Read the model definition and answer for the solid it produces. Units are mm, in the model's axes. A direction names the side the tool comes from. Give positions to 0.01 mm unless a question says otherwise; leave off trailing zeros. Write each loop counter-clockwise with the first axis right and the second up, starting at its lowest first coordinate (ties: lowest second). Pieces come first, ordered by that corner, then holes. Notation, with made-up numbers: (42, 9.25) -> (89, 9.25) arc R12 ccw to (89, 18.25) -> close; hole circle Ø4 at (-23.75, -7). An arc over 180 degrees is marked (long way). Answer as CSV lines item,"result". Start each with the question number.
1. Given pin 1 (1.6 mm diameter, centred on x = 0, y = 0, fed in from -Z); pin 2 (2 mm diameter, centred on y = -1.5, z = 12, fed in from +X), each flat-ended and moving along its own axis, determine where each tip first touches the part or whether it passes through.
2. Find the intervals of material crossed by line 1 (Y direction, x = 0, z = 3.25); line 2 (Z direction, x = 0, y = 1.5); line 3 (Z direction, x = 0, y = -1.7), in increasing order.
3. For a pull along Z with two mould halves and no side action, classify faces 1 (the flat face through (7, -3, 18)), 2 (the cylindrical face through (0.846, 0.042, 23.945)), 3 (the flat face through (0, -2, 0)) as pulls with the +Z half, pulls with the -Z half, needs draft (parallel to the pull), parting line crosses it, or undercut.
4. A tool of negligible diameter and unlimited length cuts with its end or side. For faces 4 (the cylindrical face through (-0.54, -2.44, 4.93)), 5 (the cylindrical face through (6.64, -0.04, 24.1)), from which of +Z, -Z, +X, -X, +Y, -Y can it reach the whole face along a straight path? Write none if from no direction.
5. The part is cut by section A-A, the plane x = 0. Determine the outline of the cut face in (y, z).
6. The part is cut by section C-C, the plane y = 0. Determine the outline of the cut face in (x, z), and give its area (3 significant figures).
7. The part is cut by section D-D, the plane z = 3.5. Determine the outline of the cut face in (x, y).
8. The part is cut by section B-B, the plane z = 17.5. Determine the outline of the cut face in (x, y).
from build123d import *

# Parameters (mm, degrees)
SKETCH_R        = 2.5
PAD_DEPTH       = 20
SKETCH001_R     = 1.6
POCKET_DEPTH    = 10
POCKET_FACE3_R  = 2.5
POCKET001_DEPTH = 10
SKETCH002_W     = 15
SKETCH002_H     = 15
PAD001_DEPTH    = 3
PAD002_DEPTH    = 3
SKETCH003_R     = 6.5
POCKET002_DEPTH = 6.001
FILLET_R        = 3


with BuildPart() as part:
    # Sketch → Pad (new body)
    with BuildSketch(Plane.XY):
        Circle(SKETCH_R)
    extrude(amount=PAD_DEPTH)

    # Sketch001 (on Face2 of Pad) → Pocket (cut)
    with BuildSketch(Plane(origin=(0, 0, 0), x_dir=(1, 0, 0), z_dir=(0, 0, -1))):
        Circle(SKETCH001_R)
    extrude(amount=-POCKET_DEPTH, mode=Mode.SUBTRACT)

    # Pocket Face3 → Pocket001 (cut)
    with BuildSketch(Plane(origin=(0, 0, 20), x_dir=(0, 1, 0), z_dir=(0, 0, 1))):
        Circle(POCKET_FACE3_R)
    extrude(amount=-POCKET001_DEPTH, mode=Mode.SUBTRACT)

    # Sketch002 → Pad001 (join)
    with BuildSketch(Plane.XZ):
        with Locations((0, 17.5)):
            Rectangle(SKETCH002_W, SKETCH002_H)
    extrude(amount=PAD001_DEPTH)

    # Pad001 Face5 → Pad002 (add)
    with BuildSketch(Plane(origin=(0, 0, 17.5), x_dir=(1, 0, 0), z_dir=(0, 1, 0))):
        Polygon((7.5, -7.5), (7.5, 7.5), (2.5, 7.5), (1.6, 7.5), (-1.6, 7.5), (-2.5, 7.5), (-7.5, 7.5), (-7.5, -7.5), align=None)
    extrude(amount=PAD002_DEPTH)

    # Sketch003 (on Face3 of Pad002) → Pocket002 (cut, through all)
    with BuildSketch(Plane(origin=(0, 3, 0), x_dir=(-1, 0, 0), z_dir=(0, 1, 0))):
        with Locations((0, 17.5)):
            Circle(SKETCH003_R)
    extrude(amount=-POCKET002_DEPTH, mode=Mode.SUBTRACT)

    # Fillet
    fillet_edges = [part.edges().sort_by_distance(p)[0] for p in [
        (-7.5, 0, 25),
        (-7.5, 0, 10),
        (7.5, 0, 25),
        (7.5, 0, 10),
    ]]
    fillet(fillet_edges, radius=FILLET_R)


solid = part.part
Results found:
1,pin 1,"stops at z = 10"
1,pin 2,"stops at x = 7.5"
2,line 1,"y = -2.5 to -1.6, 1.6 to 2.5"
2,line 2,"z = 10 to 11, 24 to 25"
2,line 3,"z = 0 to 11, 24 to 25"
3,face 1,"needs draft"
3,face 2,"undercut"
3,face 3,"pulls with the -Z half"
4,face 4,"-Z"
4,face 5,"+Z, +X, +Y, -Y"
5,outline,"(-3, 10) -> (-2.5, 10) -> (-2.5, 0) -> (-1.6, 0) -> (-1.6, 10) -> (1.6, 10) -> (1.6, 0) -> (2.5, 0) -> (2.5, 10) -> (3, 10) -> (3, 11) -> (-3, 11) -> close; (-3, 24) -> (3, 24) -> (3, 25) -> (-3, 25) -> close"
6,outline,"(-7.5, 13) arc R3 ccw to (-4.5, 10) -> (-2.5, 10) -> (-2.5, 0) -> (-1.6, 0) -> (-1.6, 10) -> (1.6, 10) -> (1.6, 0) -> (2.5, 0) -> (2.5, 10) -> (4.5, 10) arc R3 ccw to (7.5, 13) -> (7.5, 22) arc R3 ccw to (4.5, 25) -> (-4.5, 25) arc R3 ccw to (-7.5, 22) -> close; hole circle Ø13 at (0, 17.5)"
6,area,"103 mm²"
7,outline,"circle Ø5 at (0, 0); hole circle Ø3.2 at (0, 0)"
8,outline,"(-7.5, -3) -> (-6.5, -3) -> (-6.5, 3) -> (-7.5, 3) -> close; (6.5, -3) -> (7.5, -3) -> (7.5, 3) -> (6.5, 3) -> close"
